Here's how the part is built. I have some questions about the finished solid (model axes, mm). Face numbers are marked on the shaded views. A direction names the side the tool comes from. Give positions to 0.01 mm unless a question says otherwise; leave off trailing zeros. Write each loop counter-clockwise with the first axis right and the second up, starting at its lowest first coordinate (ties: lowest second). Pieces come first, ordered by that corner, then holes. Notation, with made-up numbers: (56, 6.25) -> (113, 6.25) arc R9 ccw to (113, 20.25) -> close; hole circle Ø3 at (-1, 61). An arc over 180 degrees is marked (long way). Put each result on its own line as item: value. Start each with the question number.
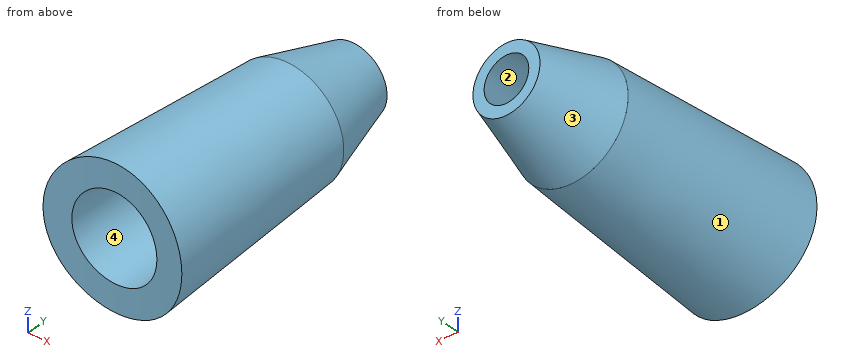
from build123d import *

# Parameters (mm, degrees)
F2_R     = 188.496796
F3_DEPTH = 25.4


with BuildPart() as f1:
    # F0 (on Top) → F1 (revolve)
    with BuildSketch(Plane.XY):
        Polygon((-19.685, 0), (-12.065, 0), (-10.795, 58.42), (-15.875, 58.42), align=None)
    revolve(axis=Axis((0, 29.21, 0), (0, -1, 0)))

    # F2 (on Top) → F3 (cut, symmetric)
    with BuildSketch(Plane.XY):
        with Locations((0, -187.268555)):
            Circle(F2_R)
    extrude(amount=F3_DEPTH, both=True, mode=Mode.SUBTRACT)

    # F4 (on Top) → F5 (revolve)
    with BuildSketch(Plane.XY):
        Polygon((-9.50494, 80.231339), (-15.875068, 58.412734), (-11.407575, 58.477067), (-6.329941, 80.231339), align=None)
    revolve(axis=Axis((0, 69.436338, 0), (0, -1, 0)))


solid = f1.part
1) I want a section at D-D, the plane y = 55. Write out the boundary of the cut face in (x, z), and give its area (3 significant figures).
2) I need wall thicknesses on probe 1 along X at (y, z) = (12, 6.5); probe 2 along X at (y, z) = (29.5, -6.5); probe 3 along Z at (x, y) = (4, 55.5). Which ranges of each line are inside material? Lowest first, please.
3) I want a section at C-C, the plane y = 38. Write out the boundary of the cut face in (x, z), and give its area (3 significant figures).
4) Thinking about a two-plate mould opening in Z: for the marked faces 1 and 2, which applies, released by +Z, released by -Z, zero draft, split by the parting line, or undercut?
5) I'm going to push flat-ended pins straight in: pin 1 Ø5 at (y, z) = (53.5, -1.5) entering from -X; pin 2 Ø1 at (y, z) = (19, 4) entering from -X; pin 3 Ø8 at (y, z) = (40, -8.5) entering from -X; pin 4 Ø15.5 at (x, z) = (2.5, 4) entering from +Y. Where does each tip first touch, or does it pass through?
6) Which directions (+Z, -Z, +X, -X, +Y, -Y) give clear straight access to the entire face, cutting with the end or side of a thin tool? Please do the marked faces 3 and 4.
Established:
1. outline: circle Ø32.2 at (0, 0); hole circle Ø21.74 at (0, 0)
1. area: 443 mm2
2. probe 1: x = -17.75 to -9.85, 9.85 to 17.75
2. probe 2: x = -16.53 to -9.39, 9.39 to 16.53
2. probe 3: z = -15.56 to -10.09, 10.09 to 15.56
3. outline: circle Ø34.41 at (0, 0); hole circle Ø22.48 at (0, 0)
3. area: 533 mm2
4. face 1: split by the parting line
4. face 2: undercut
5. pin 1: stops at x = -16.34
5. pin 2: stops at x = -18.12
5. pin 3: stops at x = -16.51
5. pin 4: stops at y = 80.23
6. face 3: +Y
6. face 4: -Y
